Build history of the part. All positions in model axes, mm. Face numbers are marked on the shaded views. A direction names the side the tool comes from. Give positions to 0.01 mm unless a question says otherwise; leave off trailing zeros. Write each loop counter-clockwise with the first axis right and the second up, starting at its lowest first coordinate (ties: lowest second). Pieces come first, ordered by that corner, then holes. Notation, with made-up numbers: (61.25, -4.75) -> (86.25, -4.75) arc R28 cw to (86.25, 16.25) -> close; hole circle Ø1 at (-27, 42.5). An arc over 180 degrees is marked (long way). Put each result on its own line as item: value.
from build123d import *

# Parameters (mm, degrees)
F0_W     = 100
F0_H     = 24
F1_DEPTH = 210
F2_W     = 98
F2_H     = 30
F2_H_2   = 16
F3_DEPTH = 26


with BuildPart() as f1:
    # F0 (on Top) → F1 (new body)
    with BuildSketch(Plane.XY):
        with Locations((-170.040163, -48.344506)):
            Rectangle(F0_W, F0_H)
    extrude(amount=-F1_DEPTH)

    # F2 (on face) → F3 (cut)
    with BuildSketch(Plane.XZ.offset(60.344506)):
        with Locations((-170.040163, -17)):
            Rectangle(F2_W, F2_H)
        with Locations((-170.040163, -49)):
            Rectangle(F2_W, F2_H)
        with Locations((-170.040163, -81)):
            Rectangle(F2_W, F2_H)
        with Locations((-170.040163, -113)):
            Rectangle(F2_W, F2_H)
        with Locations((-170.040163, -145)):
            Rectangle(F2_W, F2_H)
        with Locations((-170.040163, -177)):
            Rectangle(F2_W, F2_H)
        with Locations((-170.040163, -202)):
            Rectangle(F2_W, F2_H_2)
    extrude(amount=-F3_DEPTH, mode=Mode.SUBTRACT)


solid = f1.part
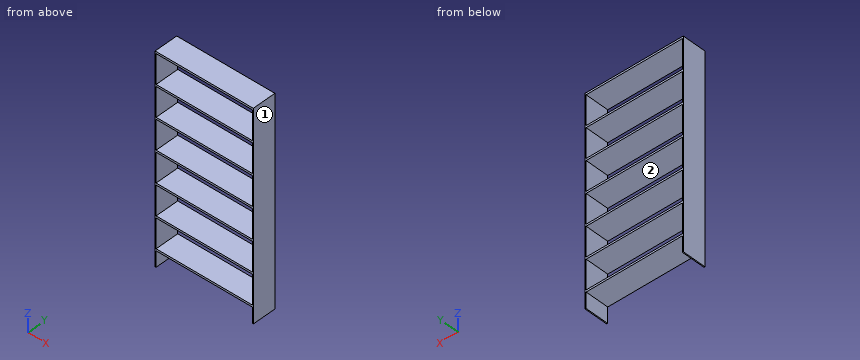
1) Pin check, flat tips, straight feed: pin 1 (6 mm diameter, centred on x = -168, y = -51.5, fed in from -Z); pin 2 (6 mm diameter, centred on x = -207.5, y = -56, fed in from +Z). Stop position of each tip, or through.
Filled sheet:
pin 1: z = -194
pin 2: z = 0
2) Slice it at B-B (x = -195.5). Write the cut outline in (y, z), plus the area to 3 significant figures.
Filled sheet:
outline: (-60.34, -194) -> (-36.34, -194) -> (-36.34, -192) -> (-60.34, -192) -> close; (-60.34, -162) -> (-36.34, -162) -> (-36.34, -160) -> (-60.34, -160) -> close; (-60.34, -130) -> (-36.34, -130) -> (-36.34, -128) -> (-60.34, -128) -> close; (-60.34, -98) -> (-36.34, -98) -> (-36.34, -96) -> (-60.34, -96) -> close; (-60.34, -66) -> (-36.34, -66) -> (-36.34, -64) -> (-60.34, -64) -> close; (-60.34, -34) -> (-36.34, -34) -> (-36.34, -32) -> (-60.34, -32) -> close; (-60.34, -2) -> (-36.34, -2) -> (-36.34, 0) -> (-60.34, 0) -> close
area: 336 mm2
3) Wall check: L1, parallel to X at y = -51.5, z = -53.5. Give the ranges that are in metal, low to high.
Filled sheet:
L1: -220.04 to -219.04, -121.04 to -120.04
4) Slice it at A-A (z = -174). Write the cut outline in (x, y), plus the area to 3 significant figures.
Filled sheet:
outline: (-220.04, -60.34) -> (-219.04, -60.34) -> (-219.04, -36.34) -> (-220.04, -36.34) -> close; (-121.04, -60.34) -> (-120.04, -60.34) -> (-120.04, -36.34) -> (-121.04, -36.34) -> close
area: 48.0 mm2
5) Slice it at C-C (y = -47). Give the number of separate pieces and of enclosed holes in the cut face, plus the area to 3 significant figures.
Filled sheet:
separate pieces: 1
enclosed holes: 6
area: 1,790 mm2
6) Tool access for the marked faces 1 and 2: list every direction of +Z, -Z, +X, -X, +Y, -Y with a clear straight run to the whole face (end or side of a thin tool).
Filled sheet:
face 1: +Z, -Z, +X, +Y, -Y
face 2: +Y, -Y
